The drawing under review shows one solid part. Ordinate dimensions are in mm from its lowest x, y, z. Coordinates: 2 decimals unless noted, no trailing zeros. Write each loop counter-clockwise with the first axis right and the second up, starting at its lowest first coordinate (ties: lowest second). Pieces come first, ordered by that corner, then holes. Notation, with made-up numbers: (-18.5, 35) - (-2.5, 35) arc R32 cw to (-2.5, 65) - close; hole circle Ø7 at (33.5, 22.25). An arc over 180 degrees is marked (long way). Use a Markdown table: item, result.
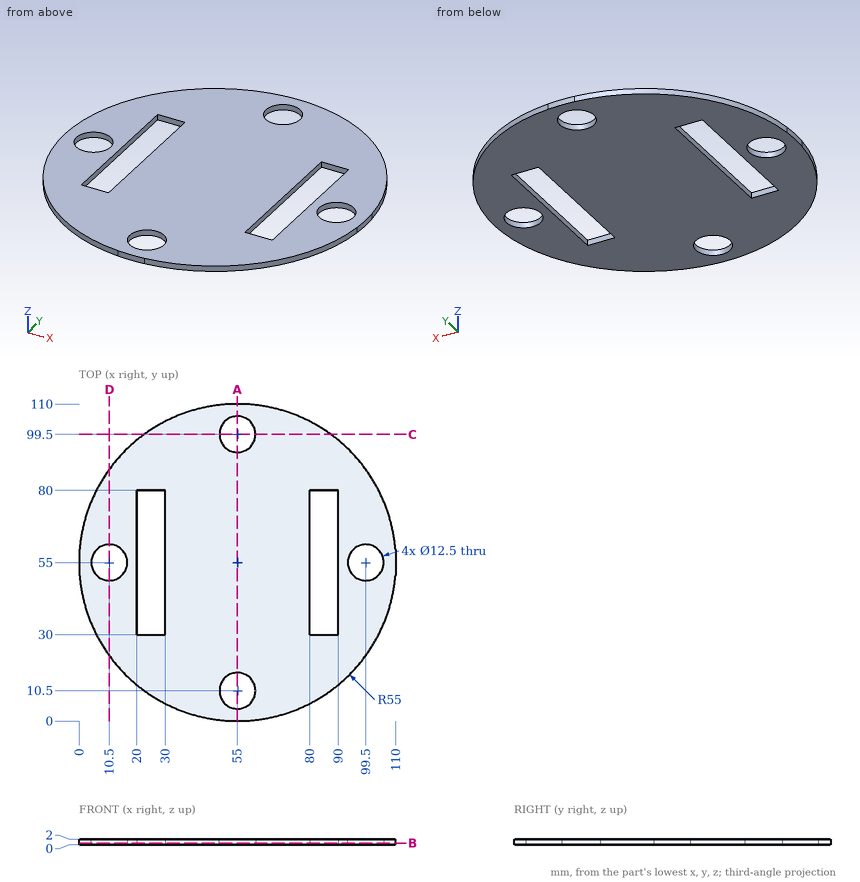
(1) For L1, parallel to X at y = 65.5, z = 1.7; L2, parallel to X at y = 75.5, z = 1.6; L3, parallel to X at y = 51.5, z = 1.3, list the stretches that pass through material, from the lowest coordinate up. Write a range as from..to.
Determined:
| item | result |
|---|---|
| L1 | 1.01..20, 30..80, 90..108.99 |
| L2 | 3.96..20, 30..80, 90..106.04 |
| L3 | 0.11..5.32, 15.68..20, 30..80, 90..94.32, 104.68..109.89 |
(2) Take a section at C-C on y = 99.5. Write out the cut boundary in (x, z), and give its area (3 significant figures).
Determined:
| item | result |
|---|---|
| outline | (22.68, 0) - (48.75, 0) - (48.75, 2) - (22.68, 2) - close; (61.25, 0) - (87.32, 0) - (87.32, 2) - (61.25, 2) - close |
| area | 104 mm2 |
(3) Take a section at B-B on z = 0.55. Write out the cut boundary in (x, y).
Determined:
| item | result |
|---|---|
| outline | circle Ø110 at (55, 55); hole circle Ø12.5 at (10.5, 55); hole (20, 30) - (30, 30) - (30, 80) - (20, 80) - close; hole circle Ø12.5 at (55, 10.5); hole circle Ø12.5 at (55, 99.5); hole (80, 30) - (90, 30) - (90, 80) - (80, 80) - close; hole circle Ø12.5 at (99.5, 55) |
(4) Take a section at A-A on x = 55. Write out the cut boundary in (y, z), and give its area (3 significant figures).
Determined:
| item | result |
|---|---|
| outline | (0, 0) - (4.25, 0) - (4.25, 2) - (0, 2) - close; (16.75, 0) - (93.25, 0) - (93.25, 2) - (16.75, 2) - close; (105.75, 0) - (110, 0) - (110, 2) - (105.75, 2) - close |
| area | 170 mm2 |
(5) For pin 1 (1 mm diameter, centred on y = 57.5, z = 1, fed in from -X); pin 2 (11 mm diameter, centred on x = 10.5, y = 55, fed in from -Z); pin 3 (1 mm diameter, centred on x = 91, z = 0.5, fed in from -Y); pin 4 (0.6 mm diameter, centred on y = 58, z = 1.5, fed in from +X), all flat-tipped, find the tip position at first contact; note any pin that passes through.
Determined:
| item | result |
|---|---|
| pin 1 | x = 0.04 |
| pin 2 | through |
| pin 3 | y = 12.99 |
| pin 4 | x = 109.93 |
